from build123d import *

# Parameters (mm, degrees)
BOSS_EXTRUDE1_DEPTH            = 6
SKETCH2_W                      = 5
SKETCH2_H                      = 130
BOSS_EXTRUDE2_DEPTH            = 24
SKETCH3_W                      = 20
SKETCH3_H                      = 12.5
CUT_EXTRUDE1_DEPTH             = 31
CBORE_FOR_M4_SHCS1_D           = 4.5
CBORE_FOR_M4_SHCS1_CBORE_D     = 8
CBORE_FOR_M4_SHCS1_CBORE_DEPTH = 4
SKETCH9_W                      = 5
SKETCH9_H                      = 20
CUT_EXTRUDE2_DEPTH             = 18
SKETCH10_W                     = 33
SKETCH10_H                     = 20
BOSS_EXTRUDE3_DEPTH            = 12
FILLET1_R                      = 5
SKETCH13_R                     = 2.5
CUT_EXTRUDE3_DEPTH             = 4.1
CHAMFER1_SIZE                  = 3
SKETCH11_R                     = 1.6
CUT_EXTRUDE4_DEPTH             = 4.5
FILLET3_R                      = 1


with BuildPart() as part:
    # Sketch1 → Boss-Extrude1 (new body)
    with BuildSketch(Plane(origin=(0, 0, 0), x_dir=(1, 0, 0), z_dir=(0, 1, 0))):
        Polygon((-25, -35), (-25, -65), (-30, -65), (-30, 65), (-25, 65), (-25, 35), (0, 35), (0, -35), align=None)
    extrude(amount=BOSS_EXTRUDE1_DEPTH)

    # Sketch2 → Boss-Extrude2 (add)
    with BuildSketch(Plane(origin=(0, 6, 0), x_dir=(1, 0, 0), z_dir=(0, 1, 0))):
        with Locations((-27.5, 0)):
            Rectangle(SKETCH2_W, SKETCH2_H)
    extrude(amount=BOSS_EXTRUDE2_DEPTH)

    # Sketch3 → Cut-Extrude1 (cut, through all)
    with BuildSketch(Plane.ZY.offset(30)):
        with Locations((-50, 6.25)):
            Rectangle(SKETCH3_W, SKETCH3_H)
        with Locations((50, 6.25)):
            Rectangle(SKETCH3_W, SKETCH3_H)
    extrude(amount=-CUT_EXTRUDE1_DEPTH, mode=Mode.SUBTRACT)

    # CBORE for M4 SHCS1 (through all)
    with Locations(Plane(origin=(0, 6, 0), x_dir=(1, 0, 0), z_dir=(0, 1, 0))):
        with Locations((-10, 15), (-10, -15)):
            CounterBoreHole(CBORE_FOR_M4_SHCS1_D / 2, CBORE_FOR_M4_SHCS1_CBORE_D / 2, CBORE_FOR_M4_SHCS1_CBORE_DEPTH)

    # Sketch9 → Cut-Extrude2 (cut)
    with BuildSketch(Plane(origin=(0, 30, 0), x_dir=(1, 0, 0), z_dir=(0, 1, 0))):
        with Locations((-27.5, 0)):
            Rectangle(SKETCH9_W, SKETCH9_H)
    extrude(amount=-CUT_EXTRUDE2_DEPTH, mode=Mode.SUBTRACT)

    # Sketch10 → Boss-Extrude3 (add, through all)
    with BuildSketch(Plane(origin=(0, 12, 0), x_dir=(1, 0, 0), z_dir=(0, 1, 0))):
        with Locations((-13.5, 0)):
            Rectangle(SKETCH10_W, SKETCH10_H)
    extrude(amount=-BOSS_EXTRUDE3_DEPTH)

    # Fillet1
    fillet1_edges = [part.edges().sort_by_distance(p)[0] for p in [
        (-27.5, 30, 10),
        (-27.5, 30, -10),
        (0, 3, -35),
        (0, 3, 35),
        (-27.5, 30, 65),
        (-27.5, 30, -65),
    ]]
    fillet(fillet1_edges, radius=FILLET1_R)

    # Sketch13 → Cut-Extrude3 (cut)
    with BuildSketch(Plane.ZY.offset(30)):
        with Locations((-20, 6)):
            Circle(SKETCH13_R)
        with Locations((20, 6)):
            Circle(SKETCH13_R)
    extrude(amount=-CUT_EXTRUDE3_DEPTH, mode=Mode.SUBTRACT)

    # Chamfer1
    chamfer1_edges = [part.edges().sort_by_distance(p)[0] for p in [
        (-30, 12, 0),
    ]]
    chamfer(chamfer1_edges, length=CHAMFER1_SIZE)

    # Sketch11 → Cut-Extrude4 (cut)
    with BuildSketch(Plane(origin=(0, 12, 0), x_dir=(1, 0, 0), z_dir=(0, 1, 0))):
        with Locations((-1.75, 3.25)):
            Circle(SKETCH11_R)
        with Locations((-1.75, -3.25)):
            Circle(SKETCH11_R)
    extrude(amount=-CUT_EXTRUDE4_DEPTH, mode=Mode.SUBTRACT)

    # Fillet3
    fillet3_edges = [part.edges().sort_by_distance(p)[0] for p in [
        (3, 6, 10),
        (3, 6, -10),
    ]]
    fillet(fillet3_edges, radius=FILLET3_R)


solid = part.part
Input: part model. Units: mm. Frame: model coordinates. A direction names the side the tool comes from. Give positions to 0.01 mm unless a question says otherwise; leave off trailing zeros. Order: outer loops, then holes, each group sorted by start corner. A loop starts at its lowest first (then second) coordinate and runs counter-clockwise, first axis right, second up. Notation, with made-up numbers: (-14, -34) -> (27, -34) arc R23 ccw to (27, -18) -> close; hole circle Ø2 at (-13.75, 41). An arc over 180 degrees is marked (long way). Use one line per item in the form item = value.
1) Mould query, pull axis Z, two halves, no side actions, for faces 1 (the cylindrical face through (-27, 29, 63)), 2 (the flat face through (-8, 2, -13)), 3 (the cylindrical face through (-27, 28, -64)), 4 (the flat face through (0, 3, 20)). Classes: pulls with the +Z half, pulls with the -Z half, needs draft (parallel to the pull), parting line crosses it, or undercut.
Response values:
face_1 = pulls with the +Z half
face_2 = undercut
face_3 = pulls with the -Z half
face_4 = needs draft
2) Section B-B, the plane x = -11. Return loops of the section in (y, z), and give its area (3 significant figures).
Response values:
outline = (0, -35) -> (6, -35) -> (6, -18.87) -> (2, -18.87) -> (2, -17.02) -> (0, -17.02) -> close; (0, -12.98) -> (2, -12.98) -> (2, -11.13) -> (6, -11.13) -> (6, -10) -> (12, -10) -> (12, 10) -> (6, 10) -> (6, 11.13) -> (2, 11.13) -> (2, 12.98) -> (0, 12.98) -> close; (0, 17.02) -> (2, 17.02) -> (2, 18.87) -> (6, 18.87) -> (6, 35) -> (0, 35) -> close
area = 462 mm^2
3) Section C-C, the plane z = 26.5. Return loops of the section in (x, y).
Response values:
outline = (-30, 0) -> (0, 0) -> (0, 6) -> (-25, 6) -> (-25, 30) -> (-30, 30) -> close
4) Line query: probe 1 along Z at (x, y) = (-10, 1.3); probe 2 along Z at (x, y) = (-10, 4.05); probe 3 along Y at (x, z) = (-28.4, 20). Output: solid intervals per line, ascending.
Response values:
probe_1 = -35 to -17.25, -12.75 to 12.75, 17.25 to 35
probe_2 = -35 to -19, -11 to 11, 19 to 35
probe_3 = 0 to 3.5, 8.5 to 30
5) First-contact query: pin 1 Ø4 at (y, z) = (6, -20) entering from +X; pin 2 Ø1.9 at (x, z) = (-1.75, -3.25) entering from +Y; pin 3 Ø3 at (y, z) = (20.5, -35.5) entering from +X. Flat tips, straight axial feed; report the tip coordinate or a pass-through.
Response values:
pin_1 = 0
pin_2 = 7.5
pin_3 = -25
6) Section D-D, the plane x = -1.75. Return loops of the section in (y, z).
Response values:
outline = (0, -33.8) -> (6, -33.8) -> (6, -10) -> (12, -10) -> (12, -4.85) -> (7.5, -4.85) -> (7.5, -1.65) -> (12, -1.65) -> (12, 1.65) -> (7.5, 1.65) -> (7.5, 4.85) -> (12, 4.85) -> (12, 10) -> (6, 10) -> (6, 33.8) -> (0, 33.8) -> close
7) Section A-A, the plane y = 17.5. Return loops of the section in (x, z).
Response values:
outline = (-30, -65) -> (-25, -65) -> (-25, -10) -> (-30, -10) -> close; (-30, 10) -> (-25, 10) -> (-25, 65) -> (-30, 65) -> close
8) Reachability of faces 5 (the cylindrical face through (-12.95, 4.03, 12.3)), 6 (the flat face through (-15, 3, 35)), 7 (the cylindrical face through (-27, 29, -12)), 8 (the flat face through (-28, 30, -38)), 9 (the flat face through (-28, 6, -40)) from +Z, -Z, +X, -X, +Y, -Y: full face, straight path, thin tool, end or side. Return the list, or none.
Response values:
face_5 = +Y
face_6 = +Z, +X, +Y, -Y
face_7 = +X, -X, +Y
face_8 = +Z, -Z, +X, -X, +Y
face_9 = +X, -X, -Y
